Input: part model. Units: mm. Frame: model coordinates. A direction names the side the tool comes from. Give positions to 0.01 mm unless a question says otherwise; leave off trailing zeros. Loops run counter-clockwise (first coordinate to the right, second up) from the corner with the lowest first, then second, coordinate; pieces in that order, holes last. Notation, with made-up numbers: M -3.5,55 L 25.5,55 A24 ccw 25.5,74 Z; hole C 63.5,-15.75 d8. An arc over 180 degrees is marked long. Return JSON: item names as keys, results as strings. Group by question number.
Autodesk Inventor part; units mm, degrees
ref_plane "YZ Plane" through (0, 0, 0) normal (1, 0, 0) x (0, 1, 0)
ref_plane "XZ Plane" through (0, 0, 0) normal (0, 1, 0) x (-1, 0, 0)
ref_plane "XY Plane" through (0, 0, 0) normal (0, 0, 1) x (1, 0, 0)
sketch "スケッチ1" plane through (0, 0, 0) normal (0, 0, 1) x (1, 0, 0)
  circle A0 centre (0, 0) radius 4.6
  dimension "d0" = 9.2
extrude "押し出し1" add sketch "スケッチ1" along normal blind 0.5
sketch "スケッチ2" plane through (0, 0, 0.5) normal (0, 0, 1) x (1, 0, 0)
  circle A0 centre (0, 0) radius 4.6
  circle A1 centre (0, 0) radius 4
  dimension "d3" = 8
extrude "押し出し2" add sketch "スケッチ2" along normal blind 2.5 contours A1
sketch "スケッチ3" plane through (0, 0, 3) normal (0, 0, 1) x (1, 0, 0)
  circle A0 centre (0, 0) radius 4
  circle A1 centre (0, 0) radius 2
  dimension "d6" = 4
hole "穴1" at (0, 0, 3) direction (0, 0, -1) diameter 4 end through all
sketch "スケッチ4" plane through (0, 0, 3) normal (0, 0, 1) x (1, 0, 0)
  circle A0 centre (0, 0) radius 4
  circle A1 centre (0, 0) radius 3.75
  circle A2 centre (0, 0) radius 2.25
  dimension "d14" = 4.5
  dimension "d15" = 7.5
extrude "押し出し3" cut sketch "スケッチ4" against normal blind 0.3 contours A1
sketch "スケッチ5" plane through (0, 0, 0) normal (0, 0, -1) x (-1, 0, 0)
  circle A0 centre (0, 0) radius 4.6
  circle A1 centre (0, 0) radius 3.75
  circle A2 centre (0, 0) radius 2.25
  dimension "d18" = 4.5
  dimension "d19" = 7.5
extrude "押し出し4" cut sketch "スケッチ5" against normal blind 0.3 contours A1
fillet "フィレット1" radius 0.1 4 edges at (2.25, 0, 0.3) (3.75, 0, 0.3) (-2.25, 0, 2.7) (-3.75, 0, 2.7)
properties part number "40" material "ステンレス鋼"
Item 1: First-contact query: pin 1 Ø1.5 at (y, z) = (-1.5, 2) entering from +X; pin 2 Ø1 at (y, z) = (2.5, 2) entering from +X. Flat tips, straight axial feed; report the tip coordinate or a pass-through.
Item 2: Section B-B, the plane x = 4.25. Return loops of the section in (y, z).
Item 3: Material intervals for line 1 (Y direction, x = 0, z = 0.15); line 2 (Y direction, x = 0, z = 1.7); line 3 (Z direction, x = -3.25, y = 1.25), sorted ascending. Write a range as from..to.
Item 4: Reachability of faces 1 (the face through (-0.867, 3.905, 1.732)), 2 (the face through (-2.4, -0.8, 0.3)), 3 (the face through (-4, 0, 0)) from +Z, -Z, +X, -X, +Y, -Y: full face, straight path, thin tool, end or side. Return the list, or none.
Item 5: Section A-A, the plane z = 2.15. Return loops of the section in (x, y).
Item 6: Pull-direction query (X, two-part tool) for faces 4 (the face through (-3.65, 2.8, 0.25)), 5 (the face through (-1.7, 3.8, 0.5)), 6 (the face through (2.4, -0.8, 2.7)); classes: pulls with the +X half, pulls with the -X half, needs draft (parallel to the pull), parting line crosses it, or undercut.
Answer below:
{
 "1": {"pin 1": "x = 3.93", "pin 2": "x = 3.46"},
 "2": {"outline": "M -1.76,0 L 1.76,0 L 1.76,0.5 L -1.76,0.5 Z"},
 "3": {"line 1": "-4.6..-3.75, -2.25..-2, 2..2.25, 3.75..4.6", "line 2": "-4..-2, 2..4", "line 3": "0.3..2.7"},
 "4": {"face 1": "+Z", "face 2": "-Z", "face 3": "-Z, +X, -X, +Y, -Y"},
 "5": {"outline": "C 0,0 d8; hole C 0,0 d4"},
 "6": {"face 4": "parting line crosses it", "face 5": "needs draft", "face 6": "undercut"}
}
